Could you check a few things on this model? Use its own coordinates, in mm. Give positions to 0.01 mm unless a question says otherwise; leave off trailing zeros. Loops run counter-clockwise (first coordinate to the right, second up) from the corner with the lowest first, then second, coordinate; pieces in that order, holes last.
1. Imagine slicing it at A-A (x = 0). List the corners of the cut face in (y, z) for me, plus the area to 3 significant figures.
2. I need wall thicknesses on line 1 along Z through (x, y) = (0, -1.25); line 2 along X through (y, z) = (-0.85, 31.5); line 3 along X through (y, z) = (-0.7, 29). Which ranges of each line are inside material? Lowest first, please.
3. Imagine slicing it at B-B (z = -13). List the corners of the cut face in (x, y) for me, plus the area to 3 significant figures.
4. Imagine slicing it at C-C (y = -1.6). Count the separate pieces of the cut face and the enclosed holes in it, plus the area to 3 significant figures.
5. For P1, Ø3.5, axis at x = -9.52, z = -19.01, coming from the -Y side, with a flat end and sliding along its axis, tell me the tip position at first contact or that it passes through.
6. Imagine slicing it at D-D (x = 10). List the corners of the cut face in (y, z) for me.
```python
from build123d import *

# Parameters (mm, degrees)
F1_DEPTH = 2.286
F3_D     = 6.5278
F5_D     = 28.575
F7_D     = 3.6576


with BuildPart() as f1:
    # F0 (on Front) → F1 (new body)
    with BuildSketch(Plane.XZ):
        with BuildLine():
            Line((25.6157214167, 42.7900233197), (-25.1842785833, 42.7900233197))
            ThreePointArc((-25.1842785833, 42.7900233197), (-29.6744066438, 40.9301513802), (-31.5342785833, 36.4400233197))
            Line((-31.5342785833, 36.4400233197), (-31.5342785833, 18.7847172783))
            ThreePointArc((-31.5342785833, 18.7847172783), (-31.3864432168, 17.422493413), (-30.9498206749, 16.1236978514))
            Line((-30.9498206749, 16.1236978514), (-14.1868850016, -20.1959961072))
            ThreePointArc((-14.1868850016, -20.1959961072), (-11.8436978478, -22.8838070833), (-8.4213429101, -23.8849766803))
            Line((-8.4213429101, -23.8849766803), (8.8527857435, -23.8849766803))
            ThreePointArc((8.8527857435, -23.8849766803), (12.2751406812, -22.8838070833), (14.6183278351, -20.1959961072))
            Line((14.6183278351, -20.1959961072), (31.3812635083, 16.1236978514))
            ThreePointArc((31.3812635083, 16.1236978514), (31.8178860502, 17.422493413), (31.9657214167, 18.7847172783))
            Line((31.9657214167, 18.7847172783), (31.9657214167, 36.4400233197))
            ThreePointArc((31.9657214167, 36.4400233197), (30.1058494773, 40.9301513802), (25.6157214167, 42.7900233197))
        make_face()
    extrude(amount=F1_DEPTH)

    # F3 (through all)
    with Locations(Plane.XZ.offset(2.286)):
        with Locations((-25.4, 30.0900233197), (0, 30.0900233197), (24.9274426514, 30.0900233197)):
            Hole(F3_D / 2)

    # F5 (through all)
    with Locations(Plane.XZ.offset(2.286)):
        with Locations((0, -3.2474766803)):
            Hole(F5_D / 2)

    # F7 (through all)
    with Locations(Plane.XZ.offset(2.286)):
        with Locations((-9.525, -19.0081766803), (9.525, -19.0081766803)):
            Hole(F7_D / 2)


solid = f1.part
```
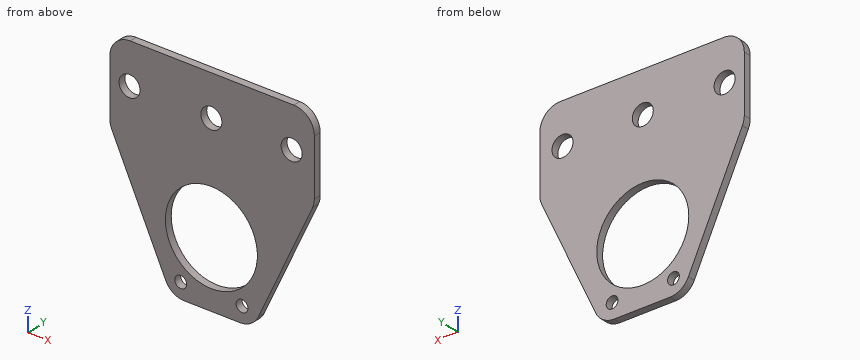
Derived:
1. outline: (-2.29, -23.88) - (0, -23.88) - (0, -17.53) - (-2.29, -17.53) - close; (-2.29, 11.04) - (0, 11.04) - (0, 26.83) - (-2.29, 26.83) - close; (-2.29, 33.35) - (0, 33.35) - (0, 42.79) - (-2.29, 42.79) - close
1. area: 72.2 mm2
2. line 1: z = -23.88 to -17.53, 11.04 to 26.83, 33.35 to 42.79
2. line 2: x = -31.53 to -28.34, -22.46 to -2.94, 2.94 to 21.98, 27.87 to 31.97
2. line 3: x = -31.53 to -28.48, -22.32 to -3.08, 3.08 to 21.85, 28 to 31.97
3. outline: (-17.51, -2.29) - (-10.44, -2.29) - (-10.44, 0) - (-17.51, 0) - close; (10.44, -2.29) - (17.94, -2.29) - (17.94, 0) - (10.44, 0) - close
3. area: 33.3 mm2
4. separate pieces: 1
4. enclosed holes: 6
4. area: 2,660 mm2
5. P1: passes through
6. outline: (-2.29, -23.78) - (0, -23.78) - (0, -20.77) - (-2.29, -20.77) - close; (-2.29, -17.24) - (0, -17.24) - (0, -13.45) - (-2.29, -13.45) - close; (-2.29, 6.96) - (0, 6.96) - (0, 42.79) - (-2.29, 42.79) - close
